Input: part model. Units: mm. Frame: model coordinates. Round coordinates to 2 decimals unless told otherwise and drop trailing zeros. Loops run counter-clockwise (first coordinate to the right, second up) from the corner with the lowest first, then second, coordinate; pieces in that order, holes last. Notation, with made-up numbers: (43.25, 24) -> (80.25, 24) arc R29 ccw to (80.25, 60) -> close; hole circle Ø2 at (-38, 73). An arc over 180 degrees is marked (long way). Answer as a JSON object with one key per item and string values. Group by question number.
Item 1: Section query A-A on z = 136.5. Return loops of the section in (x, y).
Item 2: Pin query (flat end, axial travel): pin 1 (6.5 mm diameter, centred on x = 93.57, z = -225.89, fed in from +Y); pin 2 (2 mm diameter, centred on y = 1, z = -79.5, fed in from -X); pin 3 (3 mm diameter, centred on y = -1.5, z = -111, fed in from -X); pin 4 (2 mm diameter, centred on x = -67.5, y = 0.5, fed in from -Z). Return the tip coordinate at first contact, or that it passes through.
Item 3: Section query C-C on y = 1.1. Count the separate pieces of the cut face and the enclosed holes in it, and give its area (3 significant figures).
Item 4: Section query B-B on x = -56.5. Return loops of the section in (y, z).
Item 5: Material intervals for line 1 (X direction, y = -2.55, z = -92); line 2 (X direction, y = -2.6, z = 118.5); line 3 (X direction, y = 1.8, z = 137.5), sorted ascending. Write a range as [from, to].
from build123d import *

# Parameters (mm, degrees)
SCHIZZO1_R                   = 259.5
SCHIZZO1_R_2                 = 229.5
SCHIZZO1_R_3                 = 3.5
ESTRUSIONE_ESTRUSIONE1_DEPTH = 3


with BuildPart() as part:
    # Schizzo1 → Estrusione-Estrusione1 (new, symmetric)
    with BuildSketch(Plane(origin=(0, 0, 0), x_dir=(1, 0, 0), z_dir=(0, 1, 0))):
        with Locations(Location((0, 0, 0), (0, 0, 270))):
            Circle(SCHIZZO1_R)
        with Locations(Location((0, 0, 0), (0, 0, 270))):
            Circle(SCHIZZO1_R_2, mode=Mode.SUBTRACT)
        with Locations(Location((0, 244.5, 0), (0, 0, 270))):
            Circle(SCHIZZO1_R_3, mode=Mode.SUBTRACT)
        with Locations(Location((93.566099213, 225.888545699, 0), (0, 0, 270))):
            Circle(SCHIZZO1_R_3, mode=Mode.SUBTRACT)
        with Locations(Location((172.887608, 172.887608, 0), (0, 0, 270))):
            Circle(SCHIZZO1_R_3, mode=Mode.SUBTRACT)
        with Locations(Location((225.888545699, 93.566099213, 0), (0, 0, 270))):
            Circle(SCHIZZO1_R_3, mode=Mode.SUBTRACT)
        with Locations(Location((244.5, 0, 0), (0, 0, 270))):
            Circle(SCHIZZO1_R_3, mode=Mode.SUBTRACT)
        with Locations(Location((225.888545699, -93.566099213, 0), (0, 0, 270))):
            Circle(SCHIZZO1_R_3, mode=Mode.SUBTRACT)
        with Locations(Location((172.887608, -172.887608, 0), (0, 0, 270))):
            Circle(SCHIZZO1_R_3, mode=Mode.SUBTRACT)
        with Locations(Location((93.566099213, -225.888545699, 0), (0, 0, 270))):
            Circle(SCHIZZO1_R_3, mode=Mode.SUBTRACT)
        with Locations(Location((0, -244.5, 0), (0, 0, 270))):
            Circle(SCHIZZO1_R_3, mode=Mode.SUBTRACT)
        with Locations(Location((-93.566099213, -225.888545699, 0), (0, 0, 270))):
            Circle(SCHIZZO1_R_3, mode=Mode.SUBTRACT)
        with Locations(Location((-172.887608, -172.887608, 0), (0, 0, 270))):
            Circle(SCHIZZO1_R_3, mode=Mode.SUBTRACT)
        with Locations(Location((-225.888545699, -93.566099213, 0), (0, 0, 270))):
            Circle(SCHIZZO1_R_3, mode=Mode.SUBTRACT)
        with Locations(Location((-244.5, 0, 0), (0, 0, 270))):
            Circle(SCHIZZO1_R_3, mode=Mode.SUBTRACT)
        with Locations(Location((-225.888545699, 93.566099213, 0), (0, 0, 270))):
            Circle(SCHIZZO1_R_3, mode=Mode.SUBTRACT)
        with Locations(Location((-172.887608, 172.887608, 0), (0, 0, 270))):
            Circle(SCHIZZO1_R_3, mode=Mode.SUBTRACT)
        with Locations(Location((-93.566099213, 225.888545699, 0), (0, 0, 270))):
            Circle(SCHIZZO1_R_3, mode=Mode.SUBTRACT)
    extrude(amount=ESTRUSIONE_ESTRUSIONE1_DEPTH, both=True)


solid = part.part
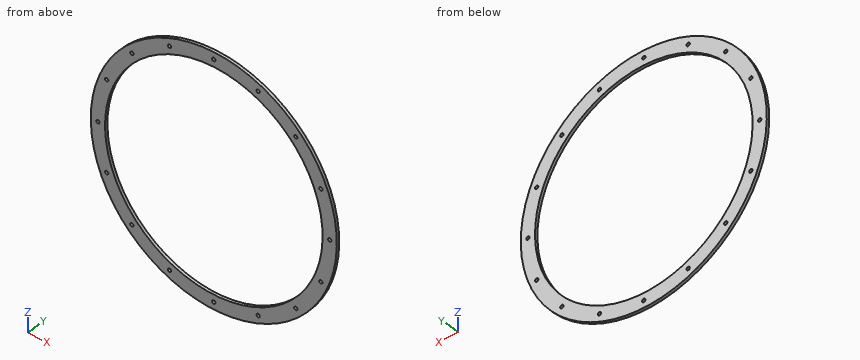
Solved:
{
 "1": {"outline": "(-220.7, -3) -> (-184.49, -3) -> (-184.49, 3) -> (-220.7, 3) -> close; (184.49, -3) -> (220.7, -3) -> (220.7, 3) -> (184.49, 3) -> close"},
 "2": {"pin 1": "through", "pin 2": "x = -247.34", "pin 3": "x = -235.27", "pin 4": "z = -250.83"},
 "3": {"separate pieces": "1", "enclosed holes": "17", "area": "45,500 mm²"},
 "4": {"outline": "(-3, -253.27) -> (3, -253.27) -> (3, -222.44) -> (-3, -222.44) -> close; (-3, 222.44) -> (3, 222.44) -> (3, 253.27) -> (-3, 253.27) -> close"},
 "5": {"line 1": "[-242.64, -229.02], [-222.76, -210.25], [210.25, 222.76], [229.02, 242.64]", "line 2": "[-230.86, -196.54], [196.54, 230.86]", "line 3": "[-220.08, -183.75], [183.75, 220.08]"}
}
